from build123d import *

# Parameters (mm, degrees)
SKETCH1_W          = 309.8
SKETCH1_H          = 270.34
BASE_FLANGE1_DEPTH = 1
FILLET1_R          = 5
SKETCH2_R          = 2.5
CUT_EXTRUDE1_DEPTH = 10
SKETCH4_R          = 7.5
CUT_EXTRUDE2_DEPTH = 10


# Sheet-metal steps are written as plain solids
with BuildPart() as part:
    # Sketch1 → Base-Flange1 (new body)
    with BuildSketch(Plane(origin=(0, 0, 0), x_dir=(1, 0, 0), z_dir=(0, 1, 0))):
        Rectangle(SKETCH1_W, SKETCH1_H)
    extrude(amount=-BASE_FLANGE1_DEPTH)

    # Fillet1
    fillet1_edges = [part.edges().sort_by_distance(p)[0] for p in [
        (-154.9, -0.5, -135.17),
        (154.9, -0.5, -135.17),
        (154.9, -0.5, 135.17),
        (-154.9, -0.5, 135.17),
    ]]
    fillet(fillet1_edges, radius=FILLET1_R)

    # Sketch2 → Cut-Extrude1 (cut)
    with BuildSketch(Plane.XZ.offset(1)):
        with Locations(Location((-141.9, 87.169485818, 0), (0, 0, 270))):
            Circle(SKETCH2_R)
        with Locations(Location((-106.9, 122.169485818, 0), (0, 0, 270))):
            Circle(SKETCH2_R)
        with Locations(Location((141.9, 87.169485818, 0), (0, 0, 90))):
            Circle(SKETCH2_R)
        with Locations(Location((106.9, 122.169485818, 0), (0, 0, 90))):
            Circle(SKETCH2_R)
        with Locations(Location((141.9, -87.169485818, 0), (0, 0, 270))):
            Circle(SKETCH2_R)
        with Locations(Location((106.9, -122.169485818, 0), (0, 0, 270))):
            Circle(SKETCH2_R)
        with Locations(Location((-141.9, -87.169485818, 0), (0, 0, 90))):
            Circle(SKETCH2_R)
        with Locations(Location((-106.9, -122.169485818, 0), (0, 0, 90))):
            Circle(SKETCH2_R)
    extrude(amount=-CUT_EXTRUDE1_DEPTH, mode=Mode.SUBTRACT)

    # Sketch4 → Cut-Extrude2 (cut)
    with BuildSketch(Plane(origin=(0, -1, 0), x_dir=(-1, 0, 0), z_dir=(0, -1, 0))):
        with Locations(Location((108.5, 75.17, 0), (0, 0, 90))):
            Circle(SKETCH4_R)
        with Locations(Location((36.166666667, 75.17, 0), (0, 0, 90))):
            Circle(SKETCH4_R)
        with Locations(Location((-36.166666667, 75.17, 0), (0, 0, 90))):
            Circle(SKETCH4_R)
        with Locations(Location((-108.5, 75.17, 0), (0, 0, 90))):
            Circle(SKETCH4_R)
    extrude(amount=-CUT_EXTRUDE2_DEPTH, mode=Mode.SUBTRACT)


solid = part.part
Here's how the part is built. I have some questions about the finished solid (model axes, mm). Coordinates: 2 decimals unless noted, no trailing zeros. Order: outer loops, then holes, each group sorted by start corner. A loop starts at its lowest first (then second) coordinate and runs counter-clockwise, first axis right, second up. Notation, with made-up numbers: (64, 52) - (111, 52) arc R32 ccw to (111, 80) - close; hole circle Ø1 at (6, -31.75). An arc over 180 degrees is marked (long way). Use CSV: the item, a comma, the result in double quotes. Start each with the question number.
1. Suppose I cut it at A-A on z = -75.17. List the corners of the cut face in (x, y) for me, then the cut area to 3 significant figures.
2. If we mould it in two halves opening along X, with no side actions, what happens to faces 1 (the face through (-2, 0, -2)), 2 (the face through (-35.837, -0.507, -67.677))? For each: +X half, -X half, draft (parallel to the pull), parting line (faces both ways), or undercut.
3. I'm going to push a flat-ended pin straight in: pin 1 (24 mm diameter, centred on x = 108.5, z = -75.17, fed in from +Y). Where does the tip first touch, or does it pass through?
4. Please list where these lines run through material, in increasing order: line 1 (X direction, y = -0.2, z = -75.17); line 2 (Z direction, x = -141.9, y = -0.7). Write a range as from..to.
Output:
1,outline,"(-154.9, -1) - (-116, -1) - (-116, 0) - (-154.9, 0) - close; (-101, -1) - (-43.67, -1) - (-43.67, 0) - (-101, 0) - close; (-28.67, -1) - (28.67, -1) - (28.67, 0) - (-28.67, 0) - close; (43.67, -1) - (101, -1) - (101, 0) - (43.67, 0) - close; (116, -1) - (154.9, -1) - (154.9, 0) - (116, 0) - close"
1,area,"250 mm2"
2,face 1,"draft"
2,face 2,"undercut"
3,pin 1,"stops at y = 0"
4,line 1,"x = -154.9..-116, -101..-43.67, -28.67..28.67, 43.67..101, 116..154.9"
4,line 2,"z = -135.17..-89.67, -84.67..84.67, 89.67..135.17"
